from build123d import *

# Parameters (mm, degrees)
F0_W     = 60
F0_H     = 100
F1_DEPTH = 10
F2_R     = 1.5
F3_DEPTH = 8
F4_R     = 1.5
F5_DEPTH = 10
F6_R     = 2.5
F7_DEPTH = 25
F8_SIZE  = 4.3
F9_R     = 3


with BuildPart() as f1:
    # F0 (on Front) → F1 (new body)
    with BuildSketch(Plane.XZ):
        Rectangle(F0_W, F0_H)
    extrude(amount=F1_DEPTH)

    # F2 (on face) → F3 (cut)
    with BuildSketch(Plane.XZ.offset(10)):
        with Locations((10, 37)):
            Circle(F2_R)
        with Locations((-10, 37)):
            Circle(F2_R)
    extrude(amount=-F3_DEPTH, mode=Mode.SUBTRACT)

    # F4 (on face) → F5 (cut)
    with BuildSketch(Plane.XY.offset(50)):
        with Locations((9, -5)):
            Circle(F4_R)
        with Locations((0, -5)):
            Circle(F4_R)
        with Locations((-9, -5)):
            Circle(F4_R)
    extrude(amount=-F5_DEPTH, mode=Mode.SUBTRACT)

    # F6 (on face) → F7 (cut)
    with BuildSketch(Plane(origin=(0, 0, 0), x_dir=(-1, 0, 0), z_dir=(0, 1, 0))):
        with Locations((0, 35)):
            Circle(F6_R)
    extrude(amount=-F7_DEPTH, mode=Mode.SUBTRACT)

    # F8
    f8_edges = [f1.edges().sort_by_distance(p)[0] for p in [
        (2.5, -10, 35),
    ]]
    chamfer(f8_edges, length=F8_SIZE)

    # F9
    f9_edges = [f1.edges().sort_by_distance(p)[0] for p in [
        (30, -5, -50),
        (-30, -5, -50),
        (-30, -5, 50),
        (30, -5, 50),
    ]]
    fillet(f9_edges, radius=F9_R)


solid = f1.part
Read the model definition and answer for the solid it produces. Units are mm, in the model's axes. A direction names the side the tool comes from. Coordinates: 2 decimals unless noted, no trailing zeros. Order: outer loops, then holes, each group sorted by start corner. A loop starts at its lowest first (then second) coordinate and runs counter-clockwise, first axis right, second up. Notation, with made-up numbers: (-26.5, 61) -> (1.5, 61) arc R10 ccw to (1.5, 67) -> close; hole circle Ø4 at (69, -38). An arc over 180 degrees is marked (long way). Answer as a JSON object with one key per item and string values.
1) Each of these flat-tipped pins is pushed along its axis until it touches: pin 1 (1.5 mm diameter, centred on x = 9.5, z = 36.5, fed in from -Y); pin 2 (6 mm diameter, centred on x = 0, z = 35, fed in from -Y); pin 3 (1.5 mm diameter, centred on x = 9.5, y = -5, fed in from +Z). Where does it stop, or does it pass through?
Model answer:
{"pin 1": "stops at y = -2", "pin 2": "stops at y = -6.2", "pin 3": "stops at z = 40"}
2) A cutting plane is placed at A-A, the plane x = 0. Determine the outline of the cut face in (y, z).
Model answer:
{"outline": "(-10, -50) -> (0, -50) -> (0, 32.5) -> (-5.7, 32.5) -> (-10, 28.2) -> close; (-10, 41.8) -> (-5.7, 37.5) -> (0, 37.5) -> (0, 50) -> (-3.5, 50) -> (-3.5, 40) -> (-6.5, 40) -> (-6.5, 50) -> (-10, 50) -> close"}
3) A tool of negligible diameter and unlimited length cuts with its end or side. For faces 4 (the face through (-10, -2, 37)), 5 (the face through (9, -5, 40)), 6 (the face through (-30, -5, -1)), from which of +Z, -Z, +X, -X, +Y, -Y can it reach the whole face along a straight path? Write none if from no direction.
Model answer:
{"face 4": "-Y", "face 5": "+Z", "face 6": "+Z, -Z, -X, +Y, -Y"}
4) The mould has two halves that part along Z. Classify faces 1 (the face through (0.54, -2.81, 32.56)), 2 (the face through (29.1, -5.07, 49.14)), 3 (the face through (-0.195, -3.513, 45.07)): released by +Z, released by -Z, zero draft, split by the parting line, or undercut.
Model answer:
{"face 1": "undercut", "face 2": "released by +Z", "face 3": "zero draft"}
5) Consider line 1 along Y through (x, z) = (0, 43); line 2 along Z through (x, y) = (10, -7.25); line 3 along Z through (x, y) = (11, -9). Determine where each line is inside the solid, lowest interval first. Write a range as from..to.
Model answer:
{"line 1": "y = -10..-6.5, -3.5..0", "line 2": "z = -50..35.5, 38.5..50", "line 3": "z = -50..35.88, 38.12..50"}
